```python
from build123d import *

# Parameters (mm, degrees)
SCHIZZO1_R                   = 6.93
ESTRUSIONE_ESTRUSIONE1_DEPTH = 103.85
ESTRUSIONE_ESTRUSIONE2_DEPTH = 1.24
SCHIZZO3_R                   = 1.495
ESTRUSIONE_ESTRUSIONE3_DEPTH = 0.88
SCHIZZO4_R                   = 3.995
ESTRUSIONE_ESTRUSIONE4_DEPTH = 15.04
SCHIZZO5_R                   = 6
ESTRUSIONE_ESTRUSIONE5_DEPTH = 28.8
TAGLIO_ESTRUSIONE1_START     = -18.82
TAGLIO_ESTRUSIONE1_DEPTH     = 18.82
SCHIZZO7_R                   = 2.5
TAGLIO_ESTRUSIONE2_DEPTH     = 107.758369227
FORO_FILETTATO_M2_5X0_45_1_D = 2.05
RACCORDO1_R                  = 1
FORO_FILETTATO_M2_5X0_45_2_D = 2.05
SCHIZZO12_R                  = 2.5
TAGLIO_ESTRUSIONE5_DEPTH     = 2.5


with BuildPart() as part:
    # Schizzo1 → Estrusione-Estrusione1 (new body)
    with BuildSketch(Plane(origin=(0, 0, 0), x_dir=(1, 0, 0), z_dir=(0, 1, 0))):
        with Locations(Location((0, 0, 0), (0, 0, 270))):
            Circle(SCHIZZO1_R)
    extrude(amount=ESTRUSIONE_ESTRUSIONE1_DEPTH)

    # Schizzo2 → Estrusione-Estrusione2 (add)
    with BuildSketch(Plane(origin=(0, 103.85, 0), x_dir=(1, 0, 0), z_dir=(0, 1, 0))):
        Polygon((-3.407809964, 1.9675), (-3.407809964, -1.9675), (0, -3.935), (3.407809964, -1.9675), (3.407809964, 1.9675), (0, 3.935), align=None)
    extrude(amount=ESTRUSIONE_ESTRUSIONE2_DEPTH)

    # Schizzo3 → Estrusione-Estrusione3 (add)
    with BuildSketch(Plane(origin=(0, 105.09, 0), x_dir=(1, 0, 0), z_dir=(0, 1, 0))):
        with Locations(Location((0, 0, 0), (0, 0, 270))):
            Circle(SCHIZZO3_R)
    extrude(amount=ESTRUSIONE_ESTRUSIONE3_DEPTH)

    # Schizzo4 → Estrusione-Estrusione4 (add)
    with BuildSketch(Plane(origin=(0, 0, 0), x_dir=(-1, 0, 0), z_dir=(0, -1, 0))):
        with Locations(Location((0, 0, 0), (0, 0, 270))):
            Circle(SCHIZZO4_R)
    extrude(amount=ESTRUSIONE_ESTRUSIONE4_DEPTH)

    # Schizzo5 → Estrusione-Estrusione5 (add)
    with BuildSketch(Plane.XZ.offset(15.04)):
        with Locations(Location((0, 0, 0), (0, 0, 270))):
            Circle(SCHIZZO5_R)
    extrude(amount=ESTRUSIONE_ESTRUSIONE5_DEPTH)

    # Schizzo6 → Taglio-Estrusione1 (cut)
    with BuildSketch(Plane.XZ.offset(43.84).offset(TAGLIO_ESTRUSIONE1_START)):
        with BuildLine():
            Line((-4.01, -4.463171518), (-4.01, 4.463171518))
            ThreePointArc((-4.01, 4.463171518), (-6, 0), (-4.01, -4.463171518))
        make_face()
        with BuildLine():
            ThreePointArc((6, 0), (5.479963504, 2.443358345), (4.01, 4.463171518))
            Line((4.01, 4.463171518), (4.01, -4.463171518))
            ThreePointArc((4.01, -4.463171518), (5.479963504, -2.443358345), (6, 0))
        make_face()
    extrude(amount=TAGLIO_ESTRUSIONE1_DEPTH, mode=Mode.SUBTRACT)

    # Schizzo7 → Taglio-Estrusione2 (cut, through all)
    with BuildSketch(Plane.ZY.offset(4.01)):
        with Locations((0, -35.84)):
            Circle(SCHIZZO7_R)
    extrude(amount=-TAGLIO_ESTRUSIONE2_DEPTH, mode=Mode.SUBTRACT)

    # Foro filettato M2.5x0.45-1 (through all)
    with Locations(Plane.ZY.offset(4.01)):
        with Locations((0, -28.34)):
            Hole(FORO_FILETTATO_M2_5X0_45_1_D / 2)

    # Raccordo1
    raccordo1_edges = [part.edges().sort_by_distance(p)[0] for p in [
        (2.1472041, -43.84, -5.602634608),
        (0, -43.84, 6),
    ]]
    fillet(raccordo1_edges, radius=RACCORDO1_R)

    # Foro filettato M2.5x0.45-2 (through all)
    with Locations(Plane(origin=(0, -40.84, 6), x_dir=(1, 0, 0), z_dir=(0, 0, 1))):
        with Locations((0, 0)):
            Hole(FORO_FILETTATO_M2_5X0_45_2_D / 2)

    # Schizzo12 → Taglio-Estrusione5 (cut)
    with BuildSketch(Plane.XY.offset(-6)):
        with Locations(Location((0, -40.84, 0), (0, 0, 233.130102354))):
            Circle(SCHIZZO12_R)
    extrude(amount=TAGLIO_ESTRUSIONE5_DEPTH, mode=Mode.SUBTRACT)


solid = part.part
```
Check sheet for the modelled part. Datum: model origin and axes. Units: mm. A direction names the side the tool comes from. Coordinates: 2 decimals unless noted, no trailing zeros. Write each loop counter-clockwise with the first axis right and the second up, starting at its lowest first coordinate (ties: lowest second). Pieces come first, ordered by that corner, then holes. Notation, with made-up numbers: (-40, 22) -> (-19, 22) arc R10 cw to (-19, 27) -> close; hole circle Ø11 at (-1.75, 74). An arc over 180 degrees is marked (long way). Use a Markdown table: item, result.
1. Release check for a two-part mould opening along Y. For faces 1 (the flat face through (-2, 105.09, 0)), 2 (the cylindrical face through (-1.627, -38.942, -4.49)), 3 (the flat face through (-4.01, -34, -2)) record: pulls with the +Y half, pulls with the -Y half, needs draft (parallel to the pull), parting line crosses it, or undercut.
Reported:
| item | result |
|---|---|
| face 1 | pulls with the +Y half |
| face 2 | undercut |
| face 3 | needs draft |
2. Tool access check on faces 4 (the flat face through (-1, -42, -3.5)), 5 (the cylindrical face through (3.9, -7.41, -0.87)), 6 (the cylindrical face through (-3.65, -25.66, 4.76)). Record the directions out of +Z, -Z, +X, -X, +Y, -Y that give a thin tool (end or side, any length) a straight path to the whole face; none if there is none.
Reported:
| item | result |
|---|---|
| face 4 | -Z |
| face 5 | none |
| face 6 | -Y |
3. Sectioned sample at A-A (y = -35.84). Enter the section's corners in (x, z), plus the area to 3 significant figures.
Reported:
| item | result |
|---|---|
| outline | (-4.01, -4.46) arc R6 ccw to (4.01, -4.46) -> (4.01, -2.5) -> (-4.01, -2.5) -> close; (-4.01, 2.5) -> (4.01, 2.5) -> (4.01, 4.46) arc R6 ccw to (-4.01, 4.46) -> close |
| area | 48.4 mm2 |
4. Scan lines: line 1 along Y through (x, z) = (0.25, 0) (3 decimals); line 2 along Y through (x, z) = (-2.25, 0) (3 decimals); line 3 along Y through (x, z) = (0, -4.8). Record each from-to range of solid material in increasing order.
Reported:
| item | result |
|---|---|
| line 1 | y = -43.84 to -41.834, -39.846 to -38.34, -33.34 to -29.365, -27.315 to 105.97 |
| line 2 | y = -43.84 to -38.34, -33.34 to -29.365, -27.315 to 105.09 |
| line 3 | y = -43.84 to -43.34, -38.34 to -15.04, 0 to 103.85 |
5. Go/stop test with flat-tipped pins: pin 1 Ø2.5 at (y, z) = (-28.34, 0) entering from -X; pin 2 Ø1 at (y, z) = (51, -4) entering from +X; pin 3 Ø2.5 at (x, y) = (0, -40.84) entering from +Z. Record where each tip stops, or that it passes through.
Reported:
| item | result |
|---|---|
| pin 1 | stops at x = -4.01 |
| pin 2 | stops at x = 5.98 |
| pin 3 | stops at z = 6 |
6. Sectioned sample at B-B (y = 28). Enter the section's corners in (x, z).
Reported:
| item | result |
|---|---|
| outline | circle Ø13.86 at (0, 0) |
